The model under review builds one solid part; all positions refer to its coordinate system, in mm. A direction names the side the tool comes from. Give positions to 0.01 mm unless a question says otherwise; leave off trailing zeros. Loops run counter-clockwise (first coordinate to the right, second up) from the corner with the lowest first, then second, coordinate; pieces in that order, holes last. Notation, with made-up numbers: M 82.5,26.25 L 102.5,26.25 A20 cw 102.5,63.25 Z; hole C 26.5,45 d10. An arc over 180 degrees is marked long. Put each result on its own line as item: value. Start each with the question number.
```python
from build123d import *

# Parameters (mm, degrees)
SKETCH1_W                = 5
SKETCH1_H                = 26.000000000000004
BOSS_EXTRUDE1_DEPTH      = 20
BOSS_EXTRUDE3_DEPTH      = 12.2
BOSS_EXTRUDE3_DEPTH_BACK = 6.5
CUT_EXTRUDE2_DEPTH       = 38.6309712869599
CUT_EXTRUDE2_DEPTH_BACK  = 38.6309712869599
SKETCH4_R                = 2.100000000000001
FILLET5_R                = 2
FILLET7_R                = 2
BOSS_EXTRUDE5_START      = 5
BOSS_EXTRUDE5_DEPTH      = 5
FILLET15_R               = 5


with BuildPart() as part:
    # Sketch1 → Boss-Extrude1 (new body)
    with BuildSketch(Plane.XY):
        Rectangle(SKETCH1_W, SKETCH1_H)
        Polygon((14.5, 13), (2.5, 13), (2.5, 5.099999999999998), (14.500000000000004, 5.099999999999999), align=None)
        Polygon((14.500000000000004, -5.099999999999999), (2.500000000000007, -5.099999999999997), (2.5, -13), (14.5, -13), align=None)
    extrude(amount=BOSS_EXTRUDE1_DEPTH)

    # Sketch3 → Boss-Extrude3 (add, two sides: drawn at the far end of the back side and taken through both)
    with BuildSketch(Plane.XY.offset(20).offset(-BOSS_EXTRUDE3_DEPTH_BACK)):
        Polygon((2.5, 13), (-14.5, 13), (-14.500000000000004, 5.099999999999999), (-2.5, 5.099999999999998), (-2.5, -5.099999999999998), (-14.500000000000004, -5.099999999999999), (-14.5, -13), (2.5, -13), align=None)
    extrude(amount=BOSS_EXTRUDE3_DEPTH + BOSS_EXTRUDE3_DEPTH_BACK)

    # Sketch4 → Cut-Extrude2 (cut, two sides: drawn at the far end of the back side and taken through both)
    with BuildSketch(Plane(origin=(0, 0, 0), x_dir=(1, 0, 0), z_dir=(0, 1, 0)).offset(-CUT_EXTRUDE2_DEPTH_BACK)):
        with Locations(Location((8.6, -10, 0), (0, 0, 270))):
            Circle(SKETCH4_R)
        with Locations(Location((-8.6, -22.85, 0), (0, 0, 270))):
            Circle(SKETCH4_R)
    extrude(amount=CUT_EXTRUDE2_DEPTH + CUT_EXTRUDE2_DEPTH_BACK, mode=Mode.SUBTRACT)

    # Fillet5
    fillet5_edges = [part.edges().sort_by_distance(p)[0] for p in [
        (14.5, 13, 10),
        (14.500000000000004, 5.099999999999999, 10),
        (2.5000000000000036, 5.099999999999998, 10),
        (2.5000000000000036, -5.099999999999997, 10),
        (14.500000000000004, -5.099999999999999, 10),
        (14.5, -13, 10),
        (-2.5, 5.099999999999998, 22.85),
        (-14.5, -13, 22.85),
        (-14.5, 13, 22.85),
        (-14.500000000000004, 5.099999999999999, 22.85),
        (-2.5, -5.099999999999998, 22.85),
        (-14.500000000000004, -5.099999999999999, 22.85),
    ]]
    fillet(fillet5_edges, radius=FILLET5_R)

    # Fillet7
    fillet7_edges = [part.edges().sort_by_distance(p)[0] for p in [
        (-2.5, 0, 0),
        (2.5, 0, 32.2),
    ]]
    fillet(fillet7_edges, radius=FILLET7_R)

    # Sketch8 → Boss-Extrude5 (add)
    with BuildSketch(Plane.XY.offset(20).offset(BOSS_EXTRUDE5_START)):
        with BuildLine():
            Line((9.21850909129393, 13), (2.5, 13))
            Line((2.5, 13), (2.5, 3.099999999999998))
            ThreePointArc((2.5, 3.099999999999998), (3.085786437626906, 4.514213562373092), (4.500000000000001, 5.099999999999998))
            Line((4.500000000000001, 5.099999999999998), (4.662191244433229, 5.099999999999998))
            ThreePointArc((4.662191244433234, 5.099999999999962), (8.333268844866092, 7.021076435787774), (10.910532200315354, 10.265311171006154))
            ThreePointArc((10.910532200315352, 10.265311171006154), (10.826416519668328, 12.104060379927068), (9.21850909129393, 13))
        make_face()
        with BuildLine():
            ThreePointArc((4.500000000000001, -5.099999999999998), (3.085786437626905, -4.514213562373093), (2.5, -3.0999999999999974))
            Line((2.5, -3.099999999999998), (2.5, -13))
            Line((2.5, -13), (9.218509091293962, -13))
            ThreePointArc((9.218509091293962, -12.999999999999998), (10.8264165196684, -12.10406037992704), (10.910532200315423, -10.265311171006077))
            ThreePointArc((10.910532200315425, -10.265311171006077), (8.33326884486619, -7.021076435787755), (4.662191244433393, -5.099999999999964))
            Line((4.662191244433386, -5.099999999999998), (4.500000000000002, -5.099999999999998))
        make_face()
    extrude(amount=-BOSS_EXTRUDE5_DEPTH)

    # Fillet15
    fillet15_edges = [part.edges().sort_by_distance(p)[0] for p in [
        (-2.5, -8.049999999999999, 13.5),
        (-2.5, 8.049999999999999, 13.5),
        (2.5, -8.049999999999999, 25),
        (2.5, 8.049999999999999, 25),
    ]]
    fillet(fillet15_edges, radius=FILLET15_R)


solid = part.part
```
Item 1: Clearance check with flat-ended pins moving along their axes: pin 1 Ø1.8 at (x, y) = (8.5, 8) entering from +Z; pin 2 Ø12 at (y, z) = (9, 7) entering from -X; pin 3 Ø1 at (y, z) = (0, 16) entering from +X. State where each tip first meets the part, or that it passes through.
Item 2: Draft analysis for pull direction Y (two halves, no side actions). For faces 1 (the flat face through (-11, 9, 13.5)), 2 (the flat face through (0, -13, 16)), 3 (the cylindrical face through (-3.07, -4.5, 20.52)), state which applies: +Y half, -Y half, draft (parallel to the pull), parting line (faces both ways), or undercut.
Item 3: Consider section C-C, the plane z = 6. Write out the cut boundary in (x, y).
Item 4: To check wall thickness, follow L1, parallel to Y at x = -10.75, z = 27.5; L2, parallel to X at y = 10.25, z = 22.85; L3, parallel to Z at x = -8.6, y = 7.25. State the ranges of each line that lie inside material, in increasing order. Write a range as [from, to].
Item 5: Consider section B-B, the plane x = -8.6. Write out the cut boundary in (y, z).
Item 6: Consider section D-D, the plane x = 8.6. Write out the cut boundary in (y, z), plus the area to 3 significant figures.
Item 7: Tool access review of faces 4 (the cylindrical face through (13.93, 5.7, 10.14)), 5 (the cylindrical face through (8.38, -7.06, 22.98)), 6 (the cylindrical face through (-13.9, -5.67, 22.98)): name each direction out of +Z, -Z, +X, -X, +Y, -Y from which nothing blocks a thin tool from reaching the whole face with its end or side.
Item 8: Consider section A-A, the plane z = 22.85. Give the number of separate pieces and of enclosed holes in the cut face, plus the area to 3 significant figures.
Report:
1. pin 1: z = 25
1. pin 2: x = -5.32
1. pin 3: x = 2.5
2. face 1: draft
2. face 2: -Y half
2. face 3: undercut
3. outline: M -2.5,-13 L 12.5,-13 A2 ccw 14.5,-11 L 14.5,-7.1 A2 ccw 12.5,-5.1 L 4.5,-5.1 A2 cw 2.5,-3.1 L 2.5,3.1 A2 cw 4.5,5.1 L 12.5,5.1 A2 ccw 14.5,7.1 L 14.5,11 A2 ccw 12.5,13 L -2.5,13 Z
4. L1: [-13, -5.1], [5.1, 13]
4. L2: [-14.5, -10.7], [-6.5, 10.9]
4. L3: [13.5, 20.75], [24.95, 32.2]
5. outline: M -13,13.5 L -5.1,13.5 L -5.1,20.75 L -13,20.75 Z; M -13,24.95 L -5.1,24.95 L -5.1,32.2 L -13,32.2 Z; M 5.1,13.5 L 13,13.5 L 13,20.75 L 5.1,20.75 Z; M 5.1,24.95 L 13,24.95 L 13,32.2 L 5.1,32.2 Z
6. outline: M -13,0 L -5.1,0 L -5.1,7.9 L -13,7.9 Z; M -13,12.1 L -5.1,12.1 L -5.1,20 L -7.25,20 L -7.25,25 L -13,25 Z; M 5.1,0 L 13,0 L 13,7.9 L 5.1,7.9 Z; M 5.1,12.1 L 13,12.1 L 13,25 L 7.25,25 L 7.25,20 L 5.1,20 Z
6. area: 307 mm²
7. face 4: +Z, -Z, +X
7. face 5: +Z, +X
7. face 6: +Z, -Z, -X
8. separate pieces: 3
8. enclosed holes: 0
8. area: 363 mm²
